```python
from build123d import *

# Parameters (mm, degrees)
EXTRUDE_1_DEPTH     = 5
SKETCH_2_R          = 5
EXTRUDE_2_DEPTH     = 11
CUT_EXTRUDE_1_REACH = 7
SKETCH_3_R          = 1.2
SKETCH_3_R_2        = 1.7
SKETCH_4_R          = 2
SKETCH_4_R_2        = 3
CUT_EXTRUDE_2_DEPTH = 2
FILLET_1_R          = 5


with BuildPart() as part:
    # 스케치1 → 보스-돌출1 (new body)
    with BuildSketch(Plane(origin=(0, 0, 0), x_dir=(1, 0, 0), z_dir=(0, 1, 0))):
        with BuildLine():
            Line((15.612494996, 12.5), (25, 12.5))
            Line((25, 12.5), (25, -12.5))
            Line((25, -12.5), (15.612494996, -12.5))
            ThreePointArc((15.612494996, -12.5), (-20, 0), (15.612494996, 12.5))
        make_face()
    extrude(amount=EXTRUDE_1_DEPTH)

    # 스케치2 → 보스-돌출2 (add)
    with BuildSketch(Plane(origin=(0, 5, 0), x_dir=(1, 0, 0), z_dir=(0, 1, 0))):
        Circle(SKETCH_2_R)
    extrude(amount=EXTRUDE_2_DEPTH)

    # 스케치3 → 컷-돌출1 (cut, up to next)
    with BuildSketch(Plane(origin=(0, 5, 0), x_dir=(1, 0, 0), z_dir=(0, 1, 0)), mode=Mode.PRIVATE) as cut_extrude_1_sk1:
        with Locations((-17.5, 0)):
            Circle(SKETCH_3_R)
    cut_extrude_1_tool1 = extrude(cut_extrude_1_sk1.sketch, amount=-CUT_EXTRUDE_1_REACH, mode=Mode.PRIVATE) & part.part
    add(cut_extrude_1_tool1.solids().sort_by_distance((-17.5, 5, 0))[0], mode=Mode.SUBTRACT)
    # 스케치3 → 컷-돌출1 (cut, up to next)
    with BuildSketch(Plane(origin=(0, 5, 0), x_dir=(1, 0, 0), z_dir=(0, 1, 0)), mode=Mode.PRIVATE) as cut_extrude_1_sk2:
        with Locations((21, 5)):
            Circle(SKETCH_3_R_2)
    cut_extrude_1_tool2 = extrude(cut_extrude_1_sk2.sketch, amount=-CUT_EXTRUDE_1_REACH, mode=Mode.PRIVATE) & part.part
    add(cut_extrude_1_tool2.solids().sort_by_distance((21, 5, -5))[0], mode=Mode.SUBTRACT)
    # 스케치3 → 컷-돌출1 (cut, up to next)
    with BuildSketch(Plane(origin=(0, 5, 0), x_dir=(1, 0, 0), z_dir=(0, 1, 0)), mode=Mode.PRIVATE) as cut_extrude_1_sk3:
        with Locations((21, -5)):
            Circle(SKETCH_3_R_2)
    cut_extrude_1_tool3 = extrude(cut_extrude_1_sk3.sketch, amount=-CUT_EXTRUDE_1_REACH, mode=Mode.PRIVATE) & part.part
    add(cut_extrude_1_tool3.solids().sort_by_distance((21, 5, 5))[0], mode=Mode.SUBTRACT)

    # 스케치4 → 컷-돌출2 (cut)
    with BuildSketch(Plane.XZ):
        with Locations((-17.5, 0)):
            Circle(SKETCH_4_R)
        with Locations((21, 5)):
            Circle(SKETCH_4_R_2)
        with Locations((21, -5)):
            Circle(SKETCH_4_R_2)
    extrude(amount=-CUT_EXTRUDE_2_DEPTH, mode=Mode.SUBTRACT)

    # 필렛1
    fillet_1_edges = [part.edges().sort_by_distance(p)[0] for p in [
        (25, 2.5, 12.5),
        (25, 2.5, -12.5),
    ]]
    fillet(fillet_1_edges, radius=FILLET_1_R)


solid = part.part
```
Work out the finished part from the listing and answer in its coordinate system (mm). A direction names the side the tool comes from. Coordinates: 2 decimals unless noted, no trailing zeros. Order: outer loops, then holes, each group sorted by start corner. A loop starts at its lowest first (then second) coordinate and runs counter-clockwise, first axis right, second up. Notation, with made-up numbers: (44.25, 74) - (67.25, 74) arc R13 cw to (67.25, 83) - close; hole circle Ø10 at (65, -37). An arc over 180 degrees is marked (long way). Answer as a JSON object with one key per item and string values.
1. Consider line 1 (Z direction, x = 21, y = 4.05); line 2 (Z direction, x = 21, y = 0.65); line 3 (Y direction, x = 14, z = -8). Determine where each line is inside the solid, lowest interval first.
Output values:
{"line 1": "z = -12.4 to -6.7, -3.3 to 3.3, 6.7 to 12.4", "line 2": "z = -12.4 to -8, -2 to 2, 8 to 12.4", "line 3": "y = 0 to 5"}
2. The mould has two halves that part along X. Classify faces 6 (the face through (23, 2, -5)), 7 (the face through (3, 5, -5)), 8 (the face through (-19.99, 2.46, 0.69)): +X half, -X half, draft (parallel to the pull), parting line (faces both ways), or undercut.
Output values:
{"face 6": "undercut", "face 7": "draft", "face 8": "parting line"}
3. Find section D-D on y = 7.25. Determine the outline of the cut face in (x, z).
Output values:
{"outline": "circle Ø10 at (0, 0)"}
4. Find section B-B on x = 21. Determine the outline of the cut face in (y, z).
Output values:
{"outline": "(0, -12.4) - (5, -12.4) - (5, -6.7) - (2, -6.7) - (2, -8) - (0, -8) - close; (0, -2) - (2, -2) - (2, -3.3) - (5, -3.3) - (5, 3.3) - (2, 3.3) - (2, 2) - (0, 2) - close; (0, 8) - (2, 8) - (2, 6.7) - (5, 6.7) - (5, 12.4) - (0, 12.4) - close"}
5. A tool of negligible diameter and unlimited length cuts with its end or side. For faces 1 (the face through (18, 2, -12.5)), 2 (the face through (23, 2, 5)), 3 (the face through (25, 2, 0)), 4 (the face through (-1.08, 10.42, 4.88)), 5 (the face through (18, 2, 12.5)), from which of +Z, -Z, +X, -X, +Y, -Y can it reach the whole face along a straight path? Write none if from no direction.
Output values:
{"face 1": "-Z, +X, +Y, -Y", "face 2": "-Y", "face 3": "+Z, -Z, +X, +Y, -Y", "face 4": "+Y", "face 5": "+Z, +X, +Y, -Y"}
6. Each of these flat-tipped pins is pushed along its axis until it touches: P1, Ø1.2, axis at x = -17, z = -0.5, coming from the -Y side; P2, Ø2, axis at x = 17.5, y = 2.5, coming from the -Z side; P3, Ø1.3, axis at x = 18, y = 3.5, coming from the +Z side. Where does it stop, or does it pass through?
Output values:
{"P1": "stops at y = 2", "P2": "stops at z = -12.5", "P3": "stops at z = 12.5"}
7. Find section C-C on x = -17.5. Determine the outline of the cut face in (y, z).
Output values:
{"outline": "(0, -9.68) - (5, -9.68) - (5, -1.2) - (2, -1.2) - (2, -2) - (0, -2) - close; (0, 2) - (2, 2) - (2, 1.2) - (5, 1.2) - (5, 9.68) - (0, 9.68) - close"}
8. Find section A-A on z = 0. Determine the outline of the cut face in (x, y), plus the area to 3 significant figures.
Output values:
{"outline": "(-20, 0) - (-19.5, 0) - (-19.5, 2) - (-18.7, 2) - (-18.7, 5) - (-20, 5) - close; (-16.3, 2) - (-15.5, 2) - (-15.5, 0) - (25, 0) - (25, 5) - (5, 5) - (5, 16) - (-5, 16) - (-5, 5) - (-16.3, 5) - close", "area": "320 mm²"}
